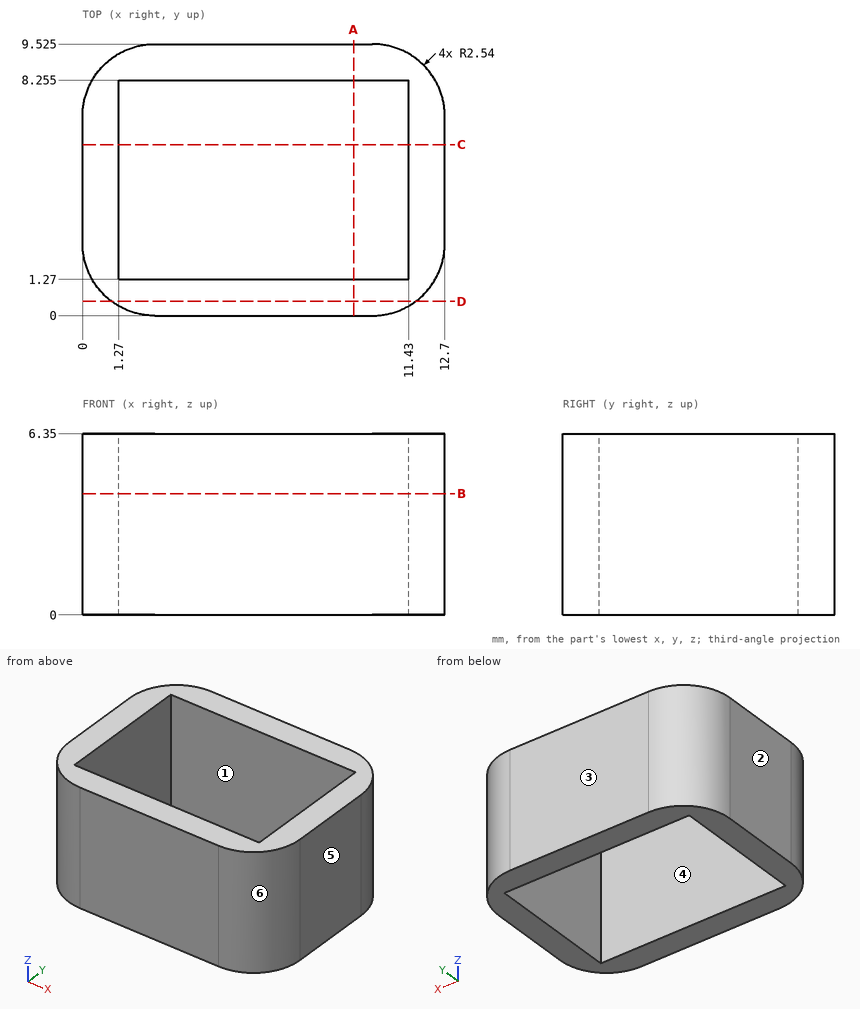
Job drawing, mm, ordinate dimensions from the low corner. One solid piece. A direction names the side the tool comes from. Give positions to 0.01 mm unless a question says otherwise; leave off trailing zeros. Order: outer loops, then holes, each group sorted by start corner. A loop starts at its lowest first (then second) coordinate and runs counter-clockwise, first axis right, second up. Notation, with made-up numbers: M -29,71.5 L 14,71.5 A18 cw 14,104.5 Z; hole C -39,-16 d7. An arc over 180 degrees is marked long. Put each result on its own line as item: value. Start each with the question number.
(1) Band-saw the part on C-C on y = 6. Give the cut face in (x, z).
(2) Pin check, flat tips, straight feed: pin 1 Ø2 at (x, z) = (8.5, 4) entering from -Y; pin 2 Ø3 at (x, y) = (3, 6) entering from -Z. Stop position of each tip, or through.
(3) Drill centre lines: L1, parallel to X at y = 3.25, z = 1.5; L2, parallel to Y at x = 3.5, z = 4 (3 decimals); L3, parallel to X at y = 7.75, z = 2.25. Where is each one in solid material? Low to high. Write a range as [from, to].
(4) Band-saw the part on A-A on x = 9.5. Give the cut face in (y, z) (3 decimals).
(5) Tool access for the marked faces 1 and 2: list every direction of +Z, -Z, +X, -X, +Y, -Y with a clear straight run to the whole face (end or side of a thin tool).
(6) Band-saw the part on B-B on z = 4.25. Give the cut face in (x, y) (3 decimals).
(7) Band-saw the part on D-D on y = 0.5. Give the cut face in (x, z).
(8) Pull direction Y, two halves, no side cores. Call the marked faces 3, 4, 5 and 6: released by +Y, released by -Y, zero draft, split by the parting line, or undercut.
Results below:
1. outline: M 0,0 L 1.27,0 L 1.27,6.35 L 0,6.35 Z; M 11.43,0 L 12.7,0 L 12.7,6.35 L 11.43,6.35 Z
2. pin 1: stops at y = 0
2. pin 2: passes through
3. L1: x = [0, 1.27], [11.43, 12.7]
3. L2: y = [0, 1.27], [8.255, 9.525]
3. L3: x = [0.12, 1.27], [11.43, 12.58]
4. outline: M 0,0 L 1.27,0 L 1.27,6.35 L 0,6.35 Z; M 8.255,0 L 9.525,0 L 9.525,6.35 L 8.255,6.35 Z
5. face 1: +Z, -Z
5. face 2: +Z, -Z, -X, +Y, -Y
6. outline: M 0,2.54 A2.54 ccw 2.54,0 L 10.16,0 A2.54 ccw 12.7,2.54 L 12.7,6.985 A2.54 ccw 10.16,9.525 L 2.54,9.525 A2.54 ccw 0,6.985 Z; hole M 1.27,1.27 L 11.43,1.27 L 11.43,8.255 L 1.27,8.255 Z
7. outline: M 1.03,0 L 11.67,0 L 11.67,6.35 L 1.03,6.35 Z
8. face 3: released by +Y
8. face 4: undercut
8. face 5: zero draft
8. face 6: released by -Y
